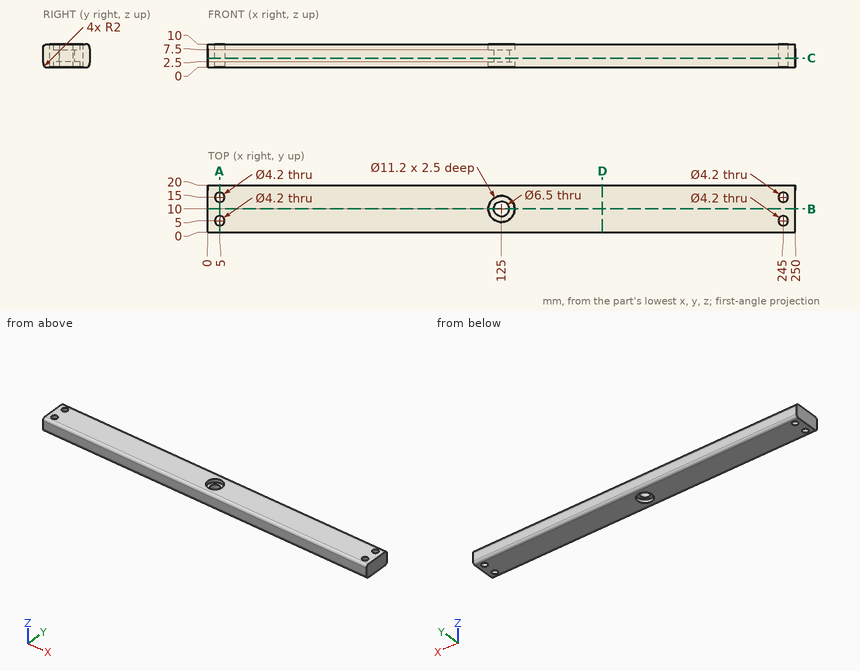
Source: three-view drawing plus pictorial views. Frame: mm from the lowest corner of the part. Coordinates: 2 decimals unless noted, no trailing zeros. Loops run counter-clockwise (first coordinate to the right, second up) from the corner with the lowest first, then second, coordinate; pieces in that order, holes last. Notation, with made-up numbers: (-24, -1) -> (14, -1) arc R19 cw to (14, 3) -> close; hole circle Ø3 at (77, 14.5). An arc over 180 degrees is marked (long way). One line per item, written item: value.
(1) Cut plane A-A (x = 5). Output: boundary loops of the cut face in (y, z).
Answer below:
outline: (0, 2) arc R2 ccw to (2, 0) -> (2.9, 0) -> (2.9, 10) -> (2, 10) arc R2 ccw to (0, 8) -> close; (7.1, 0) -> (12.9, 0) -> (12.9, 10) -> (7.1, 10) -> close; (17.1, 0) -> (18, 0) arc R2 ccw to (20, 2) -> (20, 8) arc R2 ccw to (18, 10) -> (17.1, 10) -> close
(2) Cut plane B-B (y = 10). Output: boundary loops of the cut face in (x, z), then the cut area to 3 significant figures.
Answer below:
outline: (0, 0) -> (119.4, 0) -> (119.4, 2.5) -> (121.75, 2.5) -> (121.75, 7.5) -> (119.4, 7.5) -> (119.4, 10) -> (0, 10) -> close; (128.25, 2.5) -> (130.6, 2.5) -> (130.6, 0) -> (250, 0) -> (250, 10) -> (130.6, 10) -> (130.6, 7.5) -> (128.25, 7.5) -> close
area: 2,410 mm2
(3) Ray query, line 1 along Y through (x, z) = (5, 6.5); line 2 along X through (y, z) = (10, 4.45); line 3 along Z through (x, y) = (28, 18.25). Return the intervals inside material, ascending.
Answer below:
line 1: y = 0 to 2.9, 7.1 to 12.9, 17.1 to 20
line 2: x = 0 to 121.75, 128.25 to 250
line 3: z = 0.02 to 9.98
(4) Cut plane D-D (x = 168). Output: boundary loops of the cut face in (y, z).
Answer below:
outline: (0, 2) arc R2 ccw to (2, 0) -> (18, 0) arc R2 ccw to (20, 2) -> (20, 8) arc R2 ccw to (18, 10) -> (2, 10) arc R2 ccw to (0, 8) -> close
(5) Cut plane C-C (z = 4). Output: boundary loops of the cut face in (x, y).
Answer below:
outline: (0, 0) -> (250, 0) -> (250, 20) -> (0, 20) -> close; hole circle Ø4.2 at (5, 5); hole circle Ø4.2 at (5, 15); hole circle Ø6.5 at (125, 10); hole circle Ø4.2 at (245, 5); hole circle Ø4.2 at (245, 15)
(6) Pin query (flat end, axial travel): pin 1 Ø3.5 at (x, y) = (126.5, 12) entering from -Z; pin 2 Ø9 at (x, y) = (125, 10) entering from +Z. Return the tip coordinate at first contact, or that it passes through.
Answer below:
pin 1: stops at z = 2.5
pin 2: stops at z = 7.5
